For this review, take the finished solid that the model builds, in its own axes (mm). A direction names the side the tool comes from. Round coordinates to 2 decimals unless told otherwise and drop trailing zeros. Order: outer loops, then holes, each group sorted by start corner. A loop starts at its lowest first (then second) coordinate and runs counter-clockwise, first axis right, second up. Notation, with made-up numbers: (-33.5, -28) - (-9.5, -28) arc R15 ccw to (-9.5, -8) - close; hole circle Ø9 at (65, 52). An arc over 180 degrees is marked (long way). One line per question, with ' | ' between items.
```python
from build123d import *

# Parameters (mm, degrees)
SKETCH2_W             = 45
SKETCH2_H             = 42.3
BOSS_EXTRUDE1_DEPTH   = 5
BOSS_EXTRUDE2_DEPTH   = 45
M5_CLEARANCE_HOLE1_D  = 5.5
SKETCH6_R             = 13
CUT_EXTRUDE1_DEPTH    = 5
M3_CLEARANCE_HOLE1_D  = 3.4
M5X0_8_TAPPED_HOLE1_D = 4.2


with BuildPart() as part:
    # Sketch2 → Boss-Extrude1 (new body)
    with BuildSketch(Plane(origin=(0, 0, 0), x_dir=(1, 0, 0), z_dir=(0, 1, 0))):
        Rectangle(SKETCH2_W, SKETCH2_H)
    extrude(amount=BOSS_EXTRUDE1_DEPTH)

    # Sketch3 → Boss-Extrude2 (add, through all)
    with BuildSketch(Plane(origin=(22.5, 0, 0), x_dir=(0, 0, -1), z_dir=(1, 0, 0))):
        Polygon((-21.15, 0), (-36.15, 0), (-36.15, -45), (-41.15, -45), (-41.15, 5), (-21.15, 5), align=None)
    extrude(amount=-BOSS_EXTRUDE2_DEPTH)

    # M5 Clearance Hole1 (through all)
    with Locations(Plane(origin=(0, 0, 36.15), x_dir=(-1, 0, 0), z_dir=(0, 0, -1))):
        with Locations((0, -10), (0, -25), (0, -40)):
            Hole(M5_CLEARANCE_HOLE1_D / 2)

    # Sketch6 → Cut-Extrude1 (cut)
    with BuildSketch(Plane(origin=(0, 5, 0), x_dir=(1, 0, 0), z_dir=(0, 1, 0))):
        Circle(SKETCH6_R)
    extrude(amount=-CUT_EXTRUDE1_DEPTH, mode=Mode.SUBTRACT)

    # M3 Clearance Hole1 (through all)
    with Locations(Plane(origin=(0, 5, 0), x_dir=(1, 0, 0), z_dir=(0, 1, 0))):
        with Locations((-15.5, 15.5), (-15.5, -15.5), (15.5, -15.5), (15.5, 15.5)):
            Hole(M3_CLEARANCE_HOLE1_D / 2)

    # M5x0.8 Tapped Hole1 (through all)
    with Locations(Plane(origin=(0, 5, 0), x_dir=(1, 0, 0), z_dir=(0, 1, 0))):
        with Locations((-18.25, 0), (18.25, 0)):
            Hole(M5X0_8_TAPPED_HOLE1_D / 2)


solid = part.part
```
(1) Insertion check: pin 1 (6.5 mm diameter, centred on x = 0, y = -25, fed in from +Z); pin 2 (4 mm diameter, centred on x = 15.5, z = 15.5, fed in from -Y); pin 3 (8 mm diameter, centred on x = 16, y = -9.5, fed in from -Z). Each pin has a flat end and moves straight along its axis. Give the tip position at first contact, or say it passes through.
Output values:
pin 1: z = 41.15 | pin 2: y = 0 | pin 3: z = 36.15
(2) For probe 1 along X at (y, z) = (1.3, 15.5); probe 2 along Y at (x, z) = (0, 38.15); probe 3 along Z at (x, y) = (18, 2), list the stretches that pass through material, from the lowest coordinate up. Write a range as [from, to].
Output values:
probe 1: [-22.5, -17.2], [-13.8, 13.8], [17.2, 22.5] | probe 2: [-45, -42.75], [-37.25, -27.75], [-22.25, -12.75], [-7.25, 5] | probe 3: [-21.15, -2.09], [2.09, 41.15]
(3) For faces 4 (the flat face through (0, -22, 36.15)), 5 (the cylindrical face through (13.93, 2.47, 16.15)), list the 3-axis set-ups (+Z, -Z, +X, -X, +Y, -Y) from which the entire face can be reached by the end or side of a thin tool; tool diameter is ignored.
Output values:
face 4: -Z, +X, -X, -Y | face 5: +Y, -Y
(4) We need section A-A on x = 0. State the section outline as (y, z) points.
Output values:
outline: (-45, 36.15) - (-42.75, 36.15) - (-42.75, 41.15) - (-45, 41.15) - close; (-37.25, 36.15) - (-27.75, 36.15) - (-27.75, 41.15) - (-37.25, 41.15) - close; (-22.25, 36.15) - (-12.75, 36.15) - (-12.75, 41.15) - (-22.25, 41.15) - close; (-7.25, 36.15) - (0, 36.15) - (0, 13) - (5, 13) - (5, 41.15) - (-7.25, 41.15) - close; (0, -21.15) - (5, -21.15) - (5, -13) - (0, -13) - close
(5) We need section C-C on z = -15.5. State the section outline as (x, y) points, plus the area to 3 significant figures.
Output values:
outline: (-22.5, 0) - (-17.2, 0) - (-17.2, 5) - (-22.5, 5) - close; (-13.8, 0) - (13.8, 0) - (13.8, 5) - (-13.8, 5) - close; (17.2, 0) - (22.5, 0) - (22.5, 5) - (17.2, 5) - close | area: 191 mm^2
(6) Mouldability with a two-part tool opening along X and no side actions: class faces 1 (the cylindrical face through (-17.07, 2.47, 16.15)), 2 (the flat face through (22.5, 0.5, 21.4)), 3 (the flat face through (0, 5, 17)) as released by +X, released by -X, zero draft, split by the parting line, or undercut.
Output values:
face 1: undercut | face 2: released by +X | face 3: zero draft
(7) We need section D-D on x = -18.25. State the section outline as (y, z) points.
Output values:
outline: (-45, 36.15) - (0, 36.15) - (0, 2.1) - (5, 2.1) - (5, 41.15) - (-45, 41.15) - close; (0, -21.15) - (5, -21.15) - (5, -2.1) - (0, -2.1) - close
(8) We need section B-B on z = 12. State the section outline as (x, y) points, plus the area to 3 significant figures.
Output values:
outline: (-22.5, 0) - (-5, 0) - (-5, 5) - (-22.5, 5) - close; (5, 0) - (22.5, 0) - (22.5, 5) - (5, 5) - close | area: 175 mm^2
